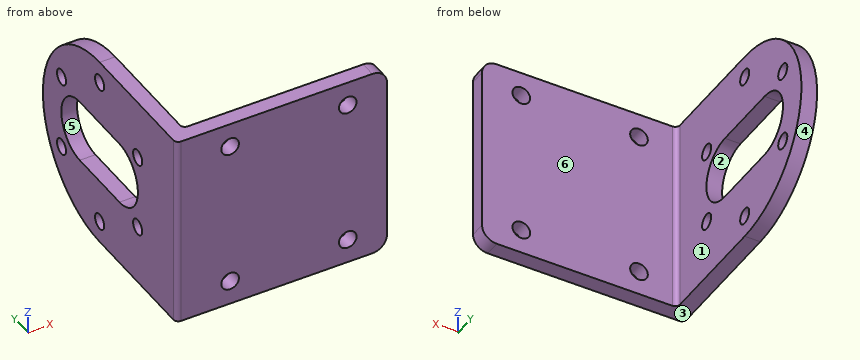
from build123d import *

# Parameters (mm, degrees)
SKETCH_1_W          = 43
SKETCH_1_H          = 40
EXTRUDE_1_DEPTH     = 3.2
SKETCH_2_W          = 3.2
SKETCH_2_H          = 40
EXTRUDE_2_DEPTH     = 23.8
EXTRUDE_3_DEPTH     = 3.2
SKETCH_4_R          = 1.8
CUT_EXTRUDE_1_DEPTH = 53.732248198
FILLET_1_R          = 3
CUT_EXTRUDE_2_REACH = 66.754
SKETCH_5_R          = 1.6
FILLET_2_R          = 1


with BuildPart() as part:
    # 草图1 → 凸台-拉伸1 (new body)
    with BuildSketch(Plane(origin=(0, 0, 0), x_dir=(1, 0, 0), z_dir=(0, 1, 0))):
        Rectangle(SKETCH_1_W, SKETCH_1_H)
    extrude(amount=EXTRUDE_1_DEPTH)

    # 草图2 → 凸台-拉伸2 (add)
    with BuildSketch(Plane(origin=(0, 3.2, 0), x_dir=(1, 0, 0), z_dir=(0, 1, 0))):
        with Locations((-19.9, 0)):
            Rectangle(SKETCH_2_W, SKETCH_2_H)
    extrude(amount=EXTRUDE_2_DEPTH)

    # 草图3 → 凸台-拉伸3 (add)
    with BuildSketch(Plane(origin=(-18.3, 0, 0), x_dir=(0, 0, -1), z_dir=(1, 0, 0))):
        with BuildLine():
            Line((-20, 27), (20, 27))
            ThreePointArc((20, 27), (0, 47), (-20, 27))
        make_face()
    extrude(amount=-EXTRUDE_3_DEPTH)

    # 草图4 → 切除-拉伸1 (cut, through all)
    with BuildSketch(Plane(origin=(0, 3.2, 0), x_dir=(1, 0, 0), z_dir=(0, 1, 0))):
        with Locations(Location((13.5, 15, 0), (0, 0, 270))):
            Circle(SKETCH_4_R)
        with Locations(Location((-10.5, 15, 0), (0, 0, 270))):
            Circle(SKETCH_4_R)
        with Locations(Location((-10.5, -15, 0), (0, 0, 270))):
            Circle(SKETCH_4_R)
        with Locations(Location((13.5, -15, 0), (0, 0, 270))):
            Circle(SKETCH_4_R)
    extrude(amount=-CUT_EXTRUDE_1_DEPTH, mode=Mode.SUBTRACT)

    # 圆角1
    fillet_1_edges = [part.edges().sort_by_distance(p)[0] for p in [
        (21.5, 1.6, 20),
        (21.5, 1.6, -20),
    ]]
    fillet(fillet_1_edges, radius=FILLET_1_R)

    # 草图5 → 切除-拉伸2 (cut, up to next)
    with BuildSketch(Plane(origin=(-18.3, 0, 0), x_dir=(0, 0, -1), z_dir=(1, 0, 0)), mode=Mode.PRIVATE) as cut_extrude_2_sk1:
        with Locations((-7.75, 40.423393759)):
            Circle(SKETCH_5_R)
    cut_extrude_2_tool1 = extrude(cut_extrude_2_sk1.sketch, amount=-CUT_EXTRUDE_2_REACH, mode=Mode.PRIVATE) & part.part
    # 草图5 → 切除-拉伸2 (cut, up to next)
    with BuildSketch(Plane(origin=(-18.3, 0, 0), x_dir=(0, 0, -1), z_dir=(1, 0, 0)), mode=Mode.PRIVATE) as cut_extrude_2_sk2:
        with Locations((7.75, 40.423393759)):
            Circle(SKETCH_5_R)
    cut_extrude_2_tool2 = extrude(cut_extrude_2_sk2.sketch, amount=-CUT_EXTRUDE_2_REACH, mode=Mode.PRIVATE) & part.part
    # 草图5 → 切除-拉伸2 (cut, up to next)
    with BuildSketch(Plane(origin=(-18.3, 0, 0), x_dir=(0, 0, -1), z_dir=(1, 0, 0)), mode=Mode.PRIVATE) as cut_extrude_2_sk3:
        with Locations((15.5, 27)):
            Circle(SKETCH_5_R)
    cut_extrude_2_tool3 = extrude(cut_extrude_2_sk3.sketch, amount=-CUT_EXTRUDE_2_REACH, mode=Mode.PRIVATE) & part.part
    # 草图5 → 切除-拉伸2 (cut, up to next)
    with BuildSketch(Plane(origin=(-18.3, 0, 0), x_dir=(0, 0, -1), z_dir=(1, 0, 0)), mode=Mode.PRIVATE) as cut_extrude_2_sk4:
        with Locations((7.75, 13.576606241)):
            Circle(SKETCH_5_R)
    cut_extrude_2_tool4 = extrude(cut_extrude_2_sk4.sketch, amount=-CUT_EXTRUDE_2_REACH, mode=Mode.PRIVATE) & part.part
    # 草图5 → 切除-拉伸2 (cut, up to next)
    with BuildSketch(Plane(origin=(-18.3, 0, 0), x_dir=(0, 0, -1), z_dir=(1, 0, 0)), mode=Mode.PRIVATE) as cut_extrude_2_sk5:
        with Locations((-7.75, 13.576606241)):
            Circle(SKETCH_5_R)
    cut_extrude_2_tool5 = extrude(cut_extrude_2_sk5.sketch, amount=-CUT_EXTRUDE_2_REACH, mode=Mode.PRIVATE) & part.part
    # 草图5 → 切除-拉伸2 (cut, up to next)
    with BuildSketch(Plane(origin=(-18.3, 0, 0), x_dir=(0, 0, -1), z_dir=(1, 0, 0)), mode=Mode.PRIVATE) as cut_extrude_2_sk6:
        with Locations((-15.5, 27)):
            Circle(SKETCH_5_R)
    cut_extrude_2_tool6 = extrude(cut_extrude_2_sk6.sketch, amount=-CUT_EXTRUDE_2_REACH, mode=Mode.PRIVATE) & part.part
    # 草图5 → 切除-拉伸2 (cut, up to next)
    with BuildSketch(Plane(origin=(-18.3, 0, 0), x_dir=(0, 0, -1), z_dir=(1, 0, 0)), mode=Mode.PRIVATE) as cut_extrude_2_sk7:
        with BuildLine():
            Line((6.5, 34), (6.5, 20))
            ThreePointArc((6.5, 20), (0, 13.5), (-6.5, 20))
            Line((-6.5, 20), (-6.5, 34))
            ThreePointArc((-6.5, 34), (0, 40.5), (6.5, 34))
        make_face()
    cut_extrude_2_tool7 = extrude(cut_extrude_2_sk7.sketch, amount=-CUT_EXTRUDE_2_REACH, mode=Mode.PRIVATE) & part.part
    add(cut_extrude_2_tool1.solids().sort_by_distance((-18.3, 40.423394, 7.75))[0], mode=Mode.SUBTRACT)
    add(cut_extrude_2_tool2.solids().sort_by_distance((-18.3, 40.423394, -7.75))[0], mode=Mode.SUBTRACT)
    add(cut_extrude_2_tool3.solids().sort_by_distance((-18.3, 27, -15.5))[0], mode=Mode.SUBTRACT)
    add(cut_extrude_2_tool4.solids().sort_by_distance((-18.3, 13.576606, -7.75))[0], mode=Mode.SUBTRACT)
    add(cut_extrude_2_tool5.solids().sort_by_distance((-18.3, 13.576606, 7.75))[0], mode=Mode.SUBTRACT)
    add(cut_extrude_2_tool6.solids().sort_by_distance((-18.3, 27, 15.5))[0], mode=Mode.SUBTRACT)
    add(cut_extrude_2_tool7.solids().sort_by_distance((-18.3, 27, 0))[0], mode=Mode.SUBTRACT)

    # 圆角2
    fillet_2_edges = [part.edges().sort_by_distance(p)[0] for p in [
        (-18.3, 3.2, 0),
        (-21.5, 0, 0),
    ]]
    fillet(fillet_2_edges, radius=FILLET_2_R)


solid = part.part
Could you check a few things on this model? Use its own coordinates, in mm. Face numbers are marked on the shaded views. A direction names the side the tool comes from. Give positions to 0.01 mm unless a question says otherwise; leave off trailing zeros. Order: outer loops, then holes, each group sorted by start corner. A loop starts at its lowest first (then second) coordinate and runs counter-clockwise, first axis right, second up.
Item 1: If we mould it in two halves opening along Z, with no side actions, what happens to the marked faces 4, 5 and 6? For each: pulls with the +Z half, pulls with the -Z half, needs draft (parallel to the pull), parting line crosses it, or undercut.
Item 2: If we section it at C-C, the plane z = 15: Write out the boundary of the cut face in (x, y), plus the area to 3 significant figures.
Item 3: For the marked faces 1, 2 and 3, which set-ups out of +Z, -Z, +X, -X, +Y, -Y let a thin tool reach every point of the face, with its end or its side?
Item 4: I need wall thicknesses on line 1 (X direction, y = 1, z = -15); line 2 (Y direction, x = -20.3, z = -7.75); line 3 (X direction, y = 19, z = 13.5). Which ranges of each line are inside material? Lowest first, please.
Item 5: I'm going to push flat-ended pins straight in: pin 1 (3.5 mm diameter, centred on x = -20, y = 30.5, fed in from -Z); pin 2 (1.9 mm diameter, centred on y = 13.58, z = -7.75, fed in from -X); pin 3 (11.5 mm diameter, centred on x = -2, z = 9, fed in from +Y); pin 4 (4 mm diameter, centred on y = 40.42, z = 7.75, fed in from +X). Where does each tip first touch, or does it pass through?
Item 6: If we section it at B-B, the plane z = 2: Write out the boundary of the cut face in (x, y).
Item 7: If we section it at A-A, the plane x = 13.5: Write out the boundary of the cut face in (y, z).
Item 8: If we section it at D-D, the plane y = 30.5: Write out the boundary of the cut face in (x, z).
Values:
1. face 4: parting line crosses it
1. face 5: undercut
1. face 6: needs draft
2. outline: (-21.5, 1) arc R1 ccw to (-20.5, 0) - (-12.3, 0) - (-12.3, 3.2) - (-17.3, 3.2) arc R1 cw to (-18.3, 4.2) - (-18.3, 25.48) - (-21.5, 25.48) - close; (-21.5, 28.52) - (-18.3, 28.52) - (-18.3, 40.23) - (-21.5, 40.23) - close; (-8.7, 0) - (11.7, 0) - (11.7, 3.2) - (-8.7, 3.2) - close; (15.3, 0) - (21.5, 0) - (21.5, 3.2) - (15.3, 3.2) - close
2. area: 223 mm2
3. face 1: +Z, -Z, +X, +Y
3. face 2: +X, -X
3. face 3: -Z, +X, -X, +Y, -Y
4. line 1: x = -21.5 to -12.3, -8.7 to 11.7, 15.3 to 21.5
4. line 2: y = 0 to 11.98, 15.18 to 38.82, 42.02 to 45.44
4. line 3: x = -21.5 to -18.3
5. pin 1: stops at z = -19.92
5. pin 2: passes through
5. pin 3: stops at y = 3.2
5. pin 4: stops at x = -18.3
6. outline: (-21.5, 1) arc R1 ccw to (-20.5, 0) - (21.5, 0) - (21.5, 3.2) - (-17.3, 3.2) arc R1 cw to (-18.3, 4.2) - (-18.3, 13.82) - (-21.5, 13.82) - close; (-21.5, 40.18) - (-18.3, 40.18) - (-18.3, 46.9) - (-21.5, 46.9) - close
7. outline: (0, -20) - (3.2, -20) - (3.2, -16.8) - (0, -16.8) - close; (0, -13.2) - (3.2, -13.2) - (3.2, 13.2) - (0, 13.2) - close; (0, 16.8) - (3.2, 16.8) - (3.2, 20) - (0, 20) - close
8. outline: (-21.5, -19.69) - (-18.3, -19.69) - (-18.3, -6.5) - (-21.5, -6.5) - close; (-21.5, 6.5) - (-18.3, 6.5) - (-18.3, 19.69) - (-21.5, 19.69) - close
